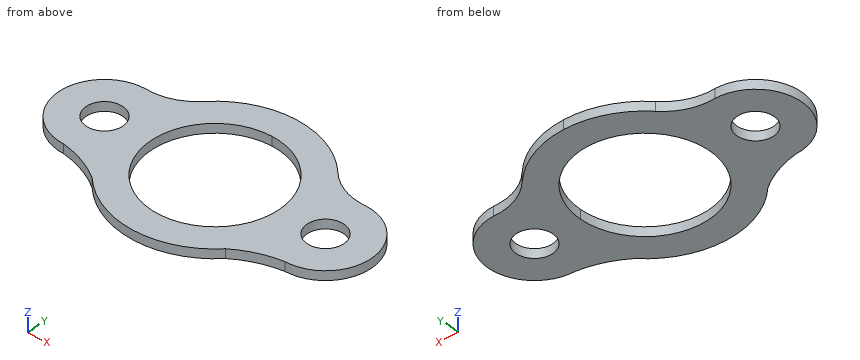
```python
from build123d import *

# Parameters (mm, degrees)
F0_R     = 12.7
F1_DEPTH = 6.35


# Not quite as in the source:
# - a feature names something its author has since deleted; it is built from what else it names


with BuildPart() as f1:
    # F0 (on Top) → F1 (new body)
    with BuildSketch(Plane.XY):
        with BuildLine():
            ThreePointArc((46.002574141, 43.7722877218), (25.0270826273, 58.3600474226), (0, 63.5))
            ThreePointArc((0, 63.5), (-25.0270826273, 58.3600474226), (-46.002574141, 43.7722877218))
            ThreePointArc((-46.002574141, 43.7722877218), (-59.7549711548, 34.379485063), (-76.2, 31.75))
            ThreePointArc((-76.2, 31.75), (-107.95, 0), (-76.2, -31.75))
            ThreePointArc((-76.2, -31.75), (-60.3918607808, -35.9792161379), (-46.002574141, -43.7722877218))
            ThreePointArc((-46.002574141, -43.7722877218), (0, -63.5), (46.002574141, -43.7722877218))
            ThreePointArc((46.002574141, -43.7722877218), (60.3918607808, -35.9792161379), (76.2, -31.75))
            ThreePointArc((76.2, -31.75), (107.95, 0), (76.2, 31.75))
            ThreePointArc((76.2, 31.75), (59.7549711548, 34.379485063), (46.002574141, 43.7722877218))
        make_face()
        with Locations((-76.2, 0)):
            Circle(F0_R, mode=Mode.SUBTRACT)
        with BuildLine():
            ThreePointArc((0, 44.45), (31.4308964237, 31.4308964237), (44.45, 0))
            ThreePointArc((44.45, 0), (-31.4308964237, -31.4308964237), (0, 44.45))
        make_face(mode=Mode.SUBTRACT)
        with Locations((76.2, 0)):
            Circle(F0_R, mode=Mode.SUBTRACT)
    extrude(amount=F1_DEPTH)


solid = f1.part
```
Could you check a few things on this model? Use its own coordinates, in mm. Round coordinates to 2 decimals unless told otherwise and drop trailing zeros. Loops run counter-clockwise (first coordinate to the right, second up) from the corner with the lowest first, then second, coordinate; pieces in that order, holes last.
Q1. I want a section at B-B (y = 7). Write out the boundary of the cut face in (x, z).
Q2. Please list where these lines run through material, in increasing order: L1, parallel to Y at x = 76.2, z = 3; L2, parallel to X at y = -5, z = 5.75.
Q3. I want a section at D-D (x = -33). Write out the boundary of the cut face in (y, z).
Q4. For P1, Ø3, axis at y = 11.5, z = 1, coming from the +X side; P2, Ø1, axis at y = -19, z = 4.5, coming from the -X side; P3, Ø2, axis at y = -2, z = 4.5, coming from the +X side, each with a flat end and sliding along its axis, tell me the tip position at first contact or that it passes through.
Q5. I want a section at C-C (x = 16). Write out the boundary of the cut face in (y, z).
Q6. I want a section at A-A (z = 4.5). Write out the boundary of the cut face in (x, y), and give its area (3 significant figures).
Answer below:
1. outline: (-107.17, 0) - (-86.8, 0) - (-86.8, 6.35) - (-107.17, 6.35) - close; (-65.6, 0) - (-43.9, 0) - (-43.9, 6.35) - (-65.6, 6.35) - close; (43.9, 0) - (65.6, 0) - (65.6, 6.35) - (43.9, 6.35) - close; (86.8, 0) - (107.17, 0) - (107.17, 6.35) - (86.8, 6.35) - close
2. L1: y = -31.75 to -12.7, 12.7 to 31.75
2. L2: x = -107.55 to -87.87, -64.53 to -44.17, 44.17 to 64.53, 87.87 to 107.55
3. outline: (-54.25, 0) - (-29.78, 0) - (-29.78, 6.35) - (-54.25, 6.35) - close; (29.78, 0) - (54.25, 0) - (54.25, 6.35) - (29.78, 6.35) - close
4. P1: stops at x = 106.33
4. P2: stops at x = -102
4. P3: stops at x = 107.93
5. outline: (-61.45, 0) - (-41.47, 0) - (-41.47, 6.35) - (-61.45, 6.35) - close; (41.47, 0) - (61.45, 0) - (61.45, 6.35) - (41.47, 6.35) - close
6. outline: (-76.2, -31.75) arc R69.81 cw to (-46, -43.77) arc R63.5 ccw to (46, -43.77) arc R69.81 cw to (76.2, -31.75) arc R31.75 ccw to (76.2, 31.75) arc R38.1 cw to (46, 43.77) arc R63.5 ccw to (-46, 43.77) arc R38.1 cw to (-76.2, 31.75) arc R31.75 ccw to start; hole circle Ø25.4 at (-76.2, 0); hole circle Ø88.9 at (0, 0); hole circle Ø25.4 at (76.2, 0)
6. area: 10,800 mm2
